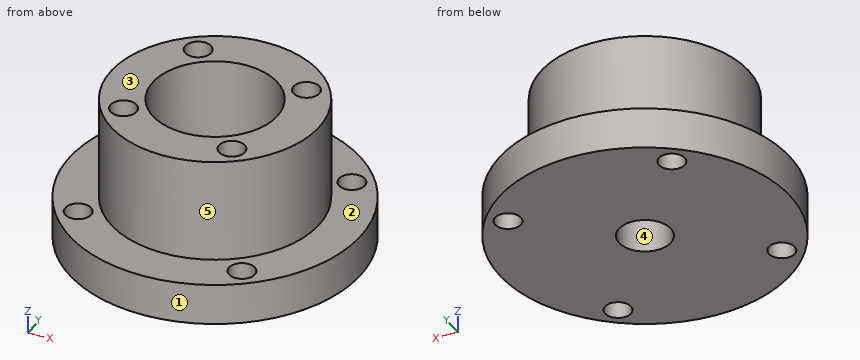
```python
from build123d import *

# Parameters (mm, degrees)
SKETCH_1_R          = 14
EXTRUDE_1_DEPTH     = 4
SKETCH_2_R          = 10
EXTRUDE_2_DEPTH     = 10
SKETCH_3_R          = 2.5
CUT_EXTRUDE_1_DEPTH = 25.248711306
SKETCH_4_R          = 6
CUT_EXTRUDE_2_DEPTH = 8
SKETCH_5_R          = 1.25
CUT_EXTRUDE_3_DEPTH = 8
SKETCH_6_R          = 1.25
CUT_EXTRUDE_4_DEPTH = 5


with BuildPart() as part:
    # 草图1 → 凸台-拉伸1 (new body)
    with BuildSketch(Plane.XY):
        Circle(SKETCH_1_R)
    extrude(amount=EXTRUDE_1_DEPTH)

    # 草图2 → 凸台-拉伸2 (add)
    with BuildSketch(Plane.XY.offset(4)):
        Circle(SKETCH_2_R)
    extrude(amount=EXTRUDE_2_DEPTH)

    # 草图3 → 切除-拉伸1 (cut, through all)
    with BuildSketch(Plane.XY.offset(14)):
        Circle(SKETCH_3_R)
    extrude(amount=-CUT_EXTRUDE_1_DEPTH, mode=Mode.SUBTRACT)

    # 草图4 → 切除-拉伸2 (cut)
    with BuildSketch(Plane.XY.offset(14)):
        Circle(SKETCH_4_R)
    extrude(amount=-CUT_EXTRUDE_2_DEPTH, mode=Mode.SUBTRACT)

    # 草图5 → 切除-拉伸3 (cut)
    with BuildSketch(Plane.XY.offset(4)):
        with Locations((-9.404150189, -7.453989484)):
            Circle(SKETCH_5_R)
        with Locations((-7.453989484, 9.404150189)):
            Circle(SKETCH_5_R)
        with Locations((9.404150189, 7.453989484)):
            Circle(SKETCH_5_R)
        with Locations((7.453989484, -9.404150189)):
            Circle(SKETCH_5_R)
    extrude(amount=-CUT_EXTRUDE_3_DEPTH, mode=Mode.SUBTRACT)

    # 草图6 → 切除-拉伸4 (cut)
    with BuildSketch(Plane.XY.offset(14)):
        with Locations((-6.326711752, -4.896194277)):
            Circle(SKETCH_6_R)
        with Locations((-4.896194277, 6.326711752)):
            Circle(SKETCH_6_R)
        with Locations((6.326711752, 4.896194277)):
            Circle(SKETCH_6_R)
        with Locations((4.896194277, -6.326711752)):
            Circle(SKETCH_6_R)
    extrude(amount=-CUT_EXTRUDE_4_DEPTH, mode=Mode.SUBTRACT)


solid = part.part
```
Geometry: final body of the model. Coordinates: model frame, mm. Face numbers are marked on the shaded views. A direction names the side the tool comes from. Give positions to 0.01 mm unless a question says otherwise; leave off trailing zeros. Loops run counter-clockwise (first coordinate to the right, second up) from the corner with the lowest first, then second, coordinate; pieces in that order, holes last. Notation, with made-up numbers: (63, -35) -> (117, -35) arc R27 cw to (117, -15) -> close; hole circle Ø2 at (-11, 8). An arc over 180 degrees is marked (long way). Return JSON: item names as keys, results as strings.
Item 1: Line query: line 1 (Y direction, x = 0, z = 10.5); line 2 (Y direction, x = 0, z = 4.25); line 3 (Y direction, x = -5, z = 10.25). Output: solid intervals per line, ascending.
Filled in:
{"line 1": "-10 to -6, 6 to 10", "line 2": "-10 to -2.5, 2.5 to 10", "line 3": "-8.66 to -3.32, 3.32 to 5.08, 7.57 to 8.66"}
Item 2: Access query for the marked faces 1 and 2. Directions: +Z, -Z, +X, -X, +Y, -Y. A direction counts if a zero-diameter tool reaches every point of the face in a straight line with its end or side. Return the directions, or none.
Filled in:
{"face 1": "+Z, -Z", "face 2": "+Z"}
Item 3: Mould query, pull axis Y, two halves, no side actions, for the marked faces 3, 4 and 5. Classes: released by +Y, released by -Y, zero draft, split by the parting line, or undercut.
Filled in:
{"face 3": "zero draft", "face 4": "undercut", "face 5": "split by the parting line"}
Item 4: Pin query (flat end, axial travel): P1, Ø6, axis at x = -4.5, z = 4, coming from the -Y side; P2, Ø2, axis at x = -7.45, y = 9.4, coming from the +Z side; P3, Ø4, axis at x = -4.5, z = 5.5, coming from the -Y side; P4, Ø6, axis at x = 5, z = 8, coming from the -Y side. Return the tip coordinate at first contact, or that it passes through.
Filled in:
{"P1": "y = -13.92", "P2": "through", "P3": "y = -13.63", "P4": "y = -9.8"}
Item 5: Section D-D, the plane y = 5.5. Output: boundary loops of the cut face in (x, z).
Filled in:
{"outline": "(-12.87, 0) -> (12.87, 0) -> (12.87, 4) -> (8.35, 4) -> (8.35, 14) -> (7.42, 14) -> (7.42, 9) -> (5.23, 9) -> (5.23, 14) -> (2.4, 14) -> (2.4, 6) -> (-2.4, 6) -> (-2.4, 14) -> (-3.96, 14) -> (-3.96, 9) -> (-5.83, 9) -> (-5.83, 14) -> (-8.35, 14) -> (-8.35, 4) -> (-12.87, 4) -> close"}
Item 6: Section A-A, the plane x = 0. Output: boundary loops of the cut face in (y, z), plus the area to 3 significant figures.
Filled in:
{"outline": "(-14, 0) -> (-2.5, 0) -> (-2.5, 6) -> (-6, 6) -> (-6, 14) -> (-10, 14) -> (-10, 4) -> (-14, 4) -> close; (2.5, 0) -> (14, 0) -> (14, 4) -> (10, 4) -> (10, 14) -> (6, 14) -> (6, 6) -> (2.5, 6) -> close", "area": "186 mm^2"}
Item 7: Section C-C, the plane z = 3.5. Output: boundary loops of the cut face in (x, y).
Filled in:
{"outline": "circle Ø28 at (0, 0); hole circle Ø2.5 at (-9.4, -7.45); hole circle Ø2.5 at (-7.45, 9.4); hole circle Ø5 at (0, 0); hole circle Ø2.5 at (7.45, -9.4); hole circle Ø2.5 at (9.4, 7.45)"}
